Geometry: final body of the model. Coordinates: model frame, mm. A direction names the side the tool comes from. Round coordinates to 2 decimals unless told otherwise and drop trailing zeros. Write each loop counter-clockwise with the first axis right and the second up, starting at its lowest first coordinate (ties: lowest second). Pieces come first, ordered by that corner, then holes.
from build123d import *

# Parameters (mm, degrees)
F1_DEPTH = 1.5875
F2_D     = 3.175


with BuildPart() as f1:
    # F0 (on Top) → F1 (new body)
    with BuildSketch(Plane.XY):
        with BuildLine():
            Line((0, 28.1305), (0, 0))
            Line((0, 0), (36.068, 0))
            Line((36.068, 0), (36.068, 42.291))
            Line((36.068, 42.291), (32.893, 42.291))
            Line((32.893, 42.291), (32.893, 45.1612))
            Line((32.893, 45.1612), (36.068, 45.1612))
            Line((36.068, 45.1612), (36.068, 49.53))
            Line((36.068, 49.53), (28.9306, 49.506645))
            ThreePointArc((28.9306, 49.506645), (22.244888, 51.383214), (17.545554, 56.495603))
            ThreePointArc((17.545554, 56.495603), (13.449123, 60.959419), (7.62, 62.611))
            Line((7.62, 62.611), (0, 62.611))
            Line((0, 62.611), (0, 34.4805))
            ThreePointArc((0, 34.4805), (2.245064, 33.550564), (3.175, 31.3055))
            ThreePointArc((3.175, 31.3055), (2.245064, 29.060436), (0, 28.1305))
        make_face()
    extrude(amount=-F1_DEPTH)

    # F2 (through all)
    with Locations(Plane.XY):
        with Locations((15.494, 51.2064), (15.6845, 35.7505), (11.1125, 9.144), (24.765, 10.6045)):
            Hole(F2_D / 2)


solid = f1.part
1) Reachability of faces 1 (the flat face through (34, 45.161, -1)), 2 (the cylindrical face through (9.6, 9.62, -0.8)) from +Z, -Z, +X, -X, +Y, -Y: full face, straight path, thin tool, end or side. Return the list, or none.
2) Section D-D on y = 43. Output: boundary loops of the cut face in (x, z), plus the area to 3 significant figures.
3) Line query: probe 1 along Y at (x, z) = (14.5, -0.95); probe 2 along Y at (x, z) = (15.5, -1.45); probe 3 along Y at (x, z) = (34.5, -0.1). Output: solid intervals per line, ascending.
4) Section B-B on z = -0.5. State how many separate pieces and enclosed holes the cut face has, plus the area to 3 significant figures.
5) Section C-C on y = 11.5. Output: boundary loops of the cut face in (x, z).
6) Section A-A on x = 2. Output: boundary loops of the cut face in (y, z), plus the area to 3 significant figures.
7) Draft query along Y for faces 3 (the flat face through (32.893, 44, -1)), 4 (the cylindrical face through (16.03, 34.2, -0.8)), 5 (the flat face through (36.068, 47, -1)), 6 (the flat face through (4, 62.611, -1)). Return one class per face: pulls with the +Y half, pulls with the -Y half, needs draft (parallel to the pull), parting line crosses it, or undercut.
Filled in:
1. face 1: +Z, -Z, +X
1. face 2: +Z, -Z
2. outline: (0, -1.59) - (32.89, -1.59) - (32.89, 0) - (0, 0) - close
2. area: 52.2 mm2
3. probe 1: y = 0 to 34.69, 36.81 to 49.97, 52.44 to 60.23
3. probe 2: y = 0 to 34.17, 37.33 to 49.62, 52.79 to 59.33
3. probe 3: y = 0 to 42.29, 45.16 to 49.52
4. separate pieces: 1
4. enclosed holes: 4
4. area: 1,960 mm2
5. outline: (0, -1.59) - (23.45, -1.59) - (23.45, 0) - (0, 0) - close; (26.08, -1.59) - (36.07, -1.59) - (36.07, 0) - (26.08, 0) - close
6. outline: (0, -1.59) - (28.84, -1.59) - (28.84, 0) - (0, 0) - close; (33.77, -1.59) - (62.61, -1.59) - (62.61, 0) - (33.77, 0) - close
6. area: 91.6 mm2
7. face 3: undercut
7. face 4: undercut
7. face 5: needs draft
7. face 6: pulls with the +Y half
